Part print with two shaded views. Sizes in mm from the minimum x, y, z corner. Coordinates: 2 decimals unless noted, no trailing zeros. Order: outer loops, then holes, each group sorted by start corner. A loop starts at its lowest first (then second) coordinate and runs counter-clockwise, first axis right, second up. Notation, with made-up numbers: (26.25, 71) - (40.25, 71) arc R20 ccw to (40.25, 90) - close; hole circle Ø4 at (-15.5, 29.5). An arc over 180 degrees is marked (long way). One line per item, written item: value.
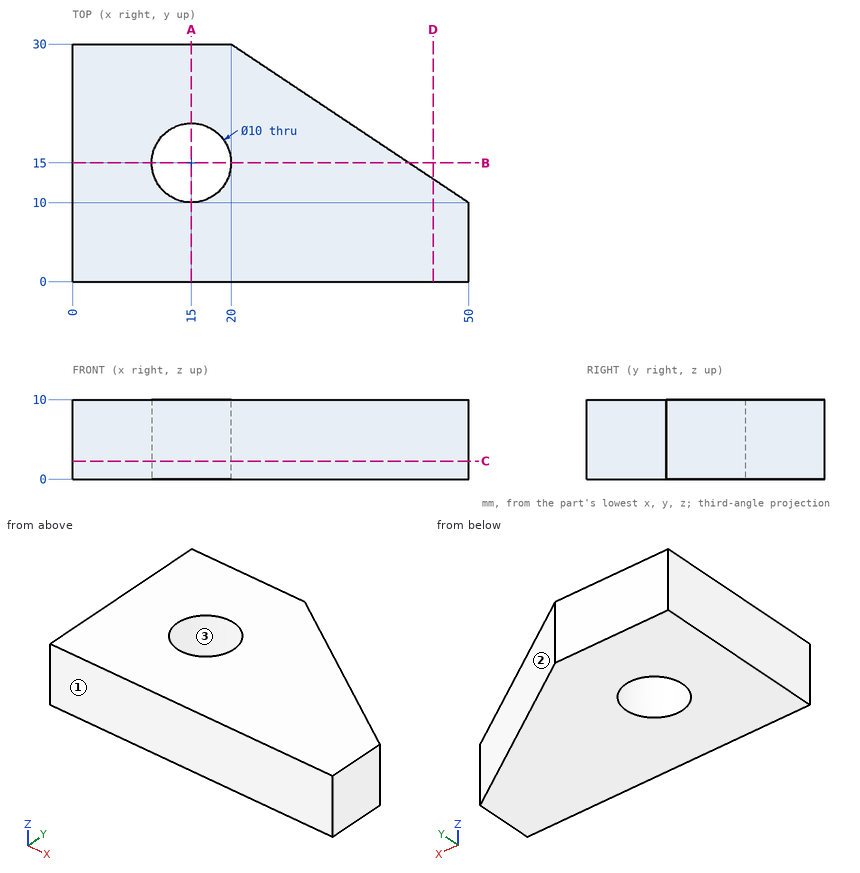
1. Probe line 1 along Y through (x, z) = (15, 4.75); line 2 along Y through (x, z) = (17.5, 5); line 3 along Y through (x, z) = (35, 8.75). List the from-to ranges inside material, lowest first.
Values found:
line 1: y = 0 to 10, 20 to 30
line 2: y = 0 to 10.67, 19.33 to 30
line 3: y = 0 to 20
2. Band-saw the part on C-C, the plane z = 2.25. Give the cut face in (x, y).
Values found:
outline: (0, 0) - (50, 0) - (50, 10) - (20, 30) - (0, 30) - close; hole circle Ø10 at (15, 15)
3. Band-saw the part on B-B, the plane y = 15. Give the cut face in (x, z), and give its area (3 significant figures).
Values found:
outline: (0, 0) - (10, 0) - (10, 10) - (0, 10) - close; (20, 0) - (42.5, 0) - (42.5, 10) - (20, 10) - close
area: 325 mm2
4. Band-saw the part on D-D, the plane x = 45.5. Give the cut face in (y, z), and give its area (3 significant figures).
Values found:
outline: (0, 0) - (13, 0) - (13, 10) - (0, 10) - close
area: 130 mm2
5. Band-saw the part on A-A, the plane x = 15. Give the cut face in (y, z), and give its area (3 significant figures).
Values found:
outline: (0, 0) - (10, 0) - (10, 10) - (0, 10) - close; (20, 0) - (30, 0) - (30, 10) - (20, 10) - close
area: 200 mm2
6. Two-plate mould, pull along Y, no slides. Class the marked faces 1, 2 and 3: pulls with the +Y half, pulls with the -Y half, needs draft (parallel to the pull), parting line crosses it, or undercut.
Values found:
face 1: pulls with the -Y half
face 2: pulls with the +Y half
face 3: undercut
7. Flat gauge pin, fed straight in: P1, Ø4, axis at y = 18.5, z = 1.5, coming from the +X side. Where does the tip first touch, or does it go through?
Values found:
P1: stops at x = 40.25
